Part model, mm, in its own coordinate system. A direction names the side the tool comes from. Round coordinates to 2 decimals unless told otherwise and drop trailing zeros. Write each loop counter-clockwise with the first axis right and the second up, starting at its lowest first coordinate (ties: lowest second). Pieces come first, ordered by that corner, then holes.
1) Saw through at B-B on y = 3.5. Write the cut outline in (x, z), and give its area (3 significant figures).
2) Saw through at D-D on z = 6.25. Write the cut outline in (x, y).
3) Flat gauge pins, fed straight in: pin 1 (6 mm diameter, centred on x = 3, z = -7, fed in from +Y); pin 2 (1.6 mm diameter, centred on y = -6, z = -0.5, fed in from -X); pin 3 (2 mm diameter, centred on x = 4.43, z = 10, fed in from -Y). Where does each tip first touch, or does it go through?
4) Drill centre lines: L1, parallel to Y at x = 6, z = 0; L2, parallel to Z at x = 7.5, y = -6.5; L3, parallel to Z at x = 1, y = 2. Where is each one in solid material? Low to high.
5) Saw through at A-A on x = 4. Write the cut outline in (y, z).
6) Saw through at C-C on x = 1. Write the cut outline in (y, z), and give its area (3 significant figures).
7) Which spindle directions (+Z, -Z, +X, -X, +Y, -Y) get a long thin tool onto all of the face, cutting with end or side? Do faces 5 (the cylindrical face through (4.056, -20.594, 10.719)), 6 (the cylindrical face through (5.566, 13.986, 9.531)), 7 (the cylindrical face through (3.042, -22.594, 12.719)). Say none if no direction does.
8) Pull direction Y, two halves, no side cores. Call faces 1 (the cylindrical face through (3.042, -22.719, -12.594)), 2 (the cylindrical face through (4.056, -2.445, -0.596)), 3 (the flat face through (7.2, 15, -0.2)), 4 (the flat face through (4, -1, -13)): +Y half, -Y half, draft (parallel to the pull), parting line (faces both ways), or undercut.
Autodesk Inventor part; units mm, degrees
ref_plane "YZ Plane" through (0, 0, 0) normal (1, 0, 0) x (0, 1, 0)
ref_plane "XZ Plane" through (0, 0, 0) normal (0, 1, 0) x (-1, 0, 0)
ref_plane "XY Plane" through (0, 0, 0) normal (0, 0, 1) x (1, 0, 0)
sketch "Sketch1" plane through (0, 0, 0) normal (1, 0, 0) x (0, 1, 0)
  line L0 (15, 15) -> (-15, 15)
  line L1 (-15, -15) -> (15, -15)
  line L2 (15, -15) -> (15, 15)
  line L3 (15, 15) -> (-15, -15) construction
  line L4 (-15, 15) -> (15, -15) construction
  line L5 (-15, -15) -> (-25, -15)
  line L6 (-25, -15) -> (-25, 15)
  line L7 (-25, 15) -> (-15, 15)
  point P0 (0, 0)
  dimension "d0" = 30
  dimension "d1" = 30
  dimension "d13" = 10
extrude "Extrusion1" add sketch "Sketch1" along normal blind 10
sketch "Sketch2" plane through (0, 0, 0) normal (-1, 0, 0) x (0, 0, 1)
  line L0 (-13, -13) -> (-13, 13)
  line L1 (13, 13) -> (13, -13)
  line L2 (13, 13) -> (-13, 13)
  line L3 (-13, -13) -> (-13, -23)
  line L4 (-13, -23) -> (13, -23)
  line L5 (13, -23) -> (13, -13)
  point P0 (0, 0)
  dimension "d14" = 10
extrude "Extrusion2" cut sketch "Sketch2" against normal blind 8
sketch "Sketch3" plane through (0, 15, 15) normal (0, 1, 0) x (1, 0, 0)
  circle A0 centre (4.4342, 15) radius 2.5
  point P0 (0, 15)
extrude "Extrusion3" add sketch "Sketch3" along normal blind 5
sketch "Sketch4" plane through (0, 13, -13) normal (0, -1, 0) x (1, 0, 0)
  circle A0 centre (4.4342, 23) radius 1.225
  circle A1 centre (4.4342, 3) radius 1.225
  point P0 (0, 13)
extrude "Extrusion4" cut sketch "Sketch4" against normal blind 2
fillet "Fillet4" radius 8 4 edges at (4, -23, 13) (4, -23, -13) (5, -25, -15) (5, -25, 15)
fillet "Fillet5" radius 4 4 edges at (10, -25, 0) (10, -22.6569, 12.6569) (10, -1, -15) (10, -22.6569, -12.6569)
sketch "Sketch11" plane through (8, 0, 0) normal (-1, 0, 0) x (0, 0, 1)
  circle A0 centre (0, -5.1293) radius 5
  circle A1 centre (0, -5.1293) radius 2.75
  point P0 (0, 0)
  dimension "d48" = 10
extrude "Extrusion13" add sketch "Sketch11" along normal blind 8
properties part number "TapaPieEfector"
Completed:
1. outline: (0, -15) - (6, -15) arc R4 ccw to (10, -11) - (10, 11) arc R4 ccw to (6, 15) - (0, 15) - (0, 13) - (8, 13) - (8, -13) - (0, -13) - close
1. area: 85.1 mm2
2. outline: (0, -25) - (6, -25) arc R4 ccw to (10, -21) - (10, 15) - (0, 15) - (0, 13) - (8, 13) - (8, -22.9) - (0, -22.9) - close
3. pin 1: stops at y = 15
3. pin 2: stops at x = 8
3. pin 3: stops at y = -24.75
4. L1: y = -25 to -23, -10.13 to -7.88, -2.38 to -0.13, 13 to 20
4. L2: z = -14.71 to -13, -4.81 to -2.38, 2.38 to 4.81, 13 to 14.71
4. L3: z = -15 to -13, 13 to 15
5. outline: (-25, -7) arc R8 ccw to (-17, -15) - (15, -15) - (15, -11.15) - (13, -11.15) - (13, -13) - (-15, -13) arc R8 cw to (-23, -5) - (-23, 5) arc R8 cw to (-15, 13) - (13, 13) - (13, 11.15) - (15, 11.15) - (15, 15) - (-17, 15) arc R8 ccw to (-25, 7) - close; circle Ø10 at (-5.13, 0); (13, -8.85) - (15, -8.85) - (15, -2.46) - (20, -2.46) - (20, 2.46) - (15, 2.46) - (15, 8.85) - (13, 8.85) - close; hole circle Ø5.5 at (-5.13, 0)
6. outline: (-25, -7) arc R8 ccw to (-17, -15) - (15, -15) - (15, 15) - (-17, 15) arc R8 ccw to (-25, 7) - close; circle Ø10 at (-5.13, 0); hole (-23, -5) arc R8 ccw to (-15, -13) - (13, -13) - (13, 13) - (-15, 13) arc R8 ccw to (-23, 5) - close; hole circle Ø5.5 at (-5.13, 0)
6. area: 319 mm2
7. face 5: -X
7. face 6: +Y
7. face 7: +Z, +X, -X, -Y
8. face 1: -Y half
8. face 2: undercut
8. face 3: +Y half
8. face 4: undercut
